For this review, take the finished solid that the model builds, in its own axes (mm). A direction names the side the tool comes from. Give positions to 0.01 mm unless a question says otherwise; leave off trailing zeros. Write each loop counter-clockwise with the first axis right and the second up, starting at its lowest first coordinate (ties: lowest second). Pieces come first, ordered by that corner, then holes. Notation, with made-up numbers: (30.25, 8) -> (40.25, 8) arc R20 cw to (40.25, 44) -> close; hole circle Ø10 at (24.25, -18.75). An arc over 180 degrees is marked (long way). Answer as CSV lines item,"result".
```python
from build123d import *

# Parameters (mm, degrees)
SKETCH1_R                = 100
BOSS_EXTRUDE1_DEPTH      = 10
SKETCH2_W                = 150
SKETCH2_H                = 150
BOSS_EXTRUDE2_DEPTH      = 20
FILLET1_R                = 20
SKETCH3_R                = 55
BOSS_EXTRUDE3_DEPTH      = 100
SKETCH4_R                = 65
BOSS_EXTRUDE4_DEPTH      = 10
SKETCH5_W                = 70
SKETCH5_H                = 90
BOSS_EXTRUDE5_DEPTH      = 90
CUT_EXTRUDE1_DEPTH       = 10
CHAMFER1_SIZE            = 10
SKETCH7_R                = 45
CUT_EXTRUDE2_DEPTH       = 100
BOSS_EXTRUDE6_DEPTH      = 10
SKETCH9_R                = 5
CUT_EXTRUDE3_DEPTH       = 2.5
FILLET9_R                = 5
CIRPATTERN1_COUNT        = 4
FILLET9_OF_CIRPATTERN1_R = 5


with BuildPart() as part:
    # Sketch1 → Boss-Extrude1 (new body)
    with BuildSketch(Plane(origin=(0, 0, 0), x_dir=(0, 0, -1), z_dir=(1, 0, 0))):
        Circle(SKETCH1_R)
    extrude(amount=BOSS_EXTRUDE1_DEPTH)

    # Sketch2 → Boss-Extrude2 (add)
    with BuildSketch(Plane(origin=(10, 0, 0), x_dir=(0, 0, -1), z_dir=(1, 0, 0))):
        Rectangle(SKETCH2_W, SKETCH2_H)
    extrude(amount=BOSS_EXTRUDE2_DEPTH)

    # Fillet1
    # the kernel refuses this fillet: 20 mm, written as the material it takes off along each edge
    with BuildSketch(Plane(origin=(10, -75, -75), x_dir=(0, 1, 0), z_dir=(1, 0, 0)), Plane(origin=(10, 75, 75), x_dir=(0, -1, 0), z_dir=(1, 0, 0)), Plane(origin=(10, -75, 75), x_dir=(0, 0, -1), z_dir=(1, 0, 0))) as fillet1_piece_1:
        with BuildLine():
            CenterArc((FILLET1_R, FILLET1_R), FILLET1_R, 180, 90)
            Line((0, FILLET1_R), (0, 0))
            Line((0, 0), (FILLET1_R, 0))
        make_face()
    extrude(amount=70, mode=Mode.SUBTRACT)
    with BuildSketch(Plane(origin=(10, 75, -75), x_dir=(0, -1, 0), z_dir=(1, 0, 0))) as fillet1_piece_2:
        with BuildLine():
            CenterArc((FILLET1_R, -FILLET1_R), FILLET1_R, 90, 90)
            Line((0, -FILLET1_R), (0, 0))
            Line((0, 0), (FILLET1_R, 0))
        make_face()
    extrude(amount=70, mode=Mode.SUBTRACT)

    # Sketch3 → Boss-Extrude3 (add)
    with BuildSketch(Plane(origin=(30, 0, 0), x_dir=(0, 0, -1), z_dir=(1, 0, 0))):
        with Locations(Location((0, 0, 0), (0, 0, 180))):
            Circle(SKETCH3_R)
    extrude(amount=BOSS_EXTRUDE3_DEPTH)

    # Sketch4 → Boss-Extrude4 (add)
    with BuildSketch(Plane(origin=(130, 0, 0), x_dir=(0, 0, -1), z_dir=(1, 0, 0))):
        Circle(SKETCH4_R)
    extrude(amount=BOSS_EXTRUDE4_DEPTH)

    # Sketch5 → Boss-Extrude5 (add)
    with BuildSketch(Plane.XY):
        with Locations((85, 0)):
            Rectangle(SKETCH5_W, SKETCH5_H)
    extrude(amount=BOSS_EXTRUDE5_DEPTH)

    # Sketch6 → Cut-Extrude1 (cut)
    with BuildSketch(Plane(origin=(120, 0, 0), x_dir=(0, 0, -1), z_dir=(1, 0, 0))):
        with BuildLine():
            Line((-90, -45), (-72.111025509, -45))
            ThreePointArc((-72.111025509, -45), (-85, 0), (-72.111025509, 45))
            Line((-72.111025509, 45), (-90, 45))
            Line((-90, 45), (-90, -45))
        make_face()
    extrude(amount=-CUT_EXTRUDE1_DEPTH, mode=Mode.SUBTRACT)

    # Chamfer1
    # the kernel refuses this chamfer: 10 mm, written as the material it adds along each edge
    with BuildSketch(Plane(origin=(110, 0, 0), x_dir=(0, -0.7581812704151473, 0.6520438337962206), z_dir=(0, -0.6520438337962206, -0.7581812704151473))) as chamfer1_piece_1_section:
        Polygon((85, -CHAMFER1_SIZE), (85 + CHAMFER1_SIZE, 0), (85, 0), align=None)
    chamfer1_piece_1 = revolve(axis=Axis((110, 0, 0), (-1, 0, 0)), revolution_arc=98.608247973, mode=Mode.PRIVATE)
    chamfer1_piece_1 = split(chamfer1_piece_1, bisect_by=Plane(origin=(118.167671654, 45, 80.674313719), z_dir=(0, -1, 0)), keep=Keep.TOP, mode=Mode.PRIVATE)
    chamfer1_piece_1 = split(chamfer1_piece_1, bisect_by=Plane(origin=(120, -31.470599687, 80.674313719), z_dir=(-1, 0, 0)), keep=Keep.TOP, mode=Mode.PRIVATE)
    chamfer1_piece_1 = split(chamfer1_piece_1, bisect_by=Plane(origin=(118.167671654, -45, 80.674313719), z_dir=(0, 1, 0)), keep=Keep.TOP, mode=Mode.PRIVATE)
    chamfer1_piece_1 = split(chamfer1_piece_1, bisect_by=Plane(origin=(118.167671654, -31.470599687, 90), z_dir=(0, 0, -1)), keep=Keep.TOP, mode=Mode.PRIVATE)
    add(chamfer1_piece_1)

    # Sketch7 → Cut-Extrude2 (cut)
    with BuildSketch(Plane(origin=(140, 0, 0), x_dir=(0, 0, -1), z_dir=(1, 0, 0))):
        Circle(SKETCH7_R)
    extrude(amount=-CUT_EXTRUDE2_DEPTH, mode=Mode.SUBTRACT)

    # Sketch8 → Boss-Extrude6 (add)
    with BuildSketch(Plane(origin=(30, 0, 0), x_dir=(0, 0, -1), z_dir=(1, 0, 0))):
        Polygon((67.320508076, -61.627449546), (67.320508076, -51.627449546), (58.660254038, -46.627449546), (50, -51.627449546), (50, -61.627449546), (58.660254038, -66.627449546), align=None)
    boss_extrude6 = extrude(amount=BOSS_EXTRUDE6_DEPTH)

    # Sketch9 → Cut-Extrude3 (cut)
    with BuildSketch(Plane(origin=(40, 0, 0), x_dir=(0, 0, -1), z_dir=(1, 0, 0))):
        with Locations((58.588222401, -56.525256823)):
            Circle(SKETCH9_R)
    cut_extrude3 = extrude(amount=-CUT_EXTRUDE3_DEPTH, mode=Mode.SUBTRACT)

    # Fillet9
    # the kernel refuses this fillet: 5 mm, written as the material it adds along each edge
    with BuildSketch(Plane(origin=(37.5, -56.525256823, -58.588222401), x_dir=(0, 0, -1), z_dir=(0, -1, 0))) as fillet9_piece_1:
        with BuildLine():
            CenterArc((0.669872981, 5), FILLET9_R, 270, 60)
            Line((0.669872981, 0), (0.669872981, -0.1))
            Line((0.669872981, -0.1), (5, -0.1))
            Line((5, -0.1), (5.1, 0))
            ThreePointArc((5.1, 0), (5.1, 1.25), (5.08660254, 2.45))
            Line((5.08660254, 2.45), (5, 2.5))
        make_face()
    revolve(axis=Axis((37.5, -56.525256823, -58.588222401), (1, 0, 0)))

    # CirPattern1: Boss-Extrude6, Cut-Extrude3 ×4 about axis
    cirpattern1_axis = Axis((0, 0, 0), (1, 0, 0))
    add([boss_extrude6.rotate(cirpattern1_axis, i * 360 / CIRPATTERN1_COUNT) for i in range(1, CIRPATTERN1_COUNT)])
    add([cut_extrude3.rotate(cirpattern1_axis, i * 360 / CIRPATTERN1_COUNT) for i in range(1, CIRPATTERN1_COUNT)], mode=Mode.SUBTRACT)

    # Fillet9 of CirPattern1
    # the kernel refuses this fillet: 5 mm, written as the material it adds along each edge
    with BuildSketch(Plane(origin=(37.5, 58.588222401, -56.525256823), x_dir=(0, 1, 0), z_dir=(0, 0, -1))) as fillet9_of_cirpattern1_piece_1:
        with BuildLine():
            CenterArc((0.669872981, 5), FILLET9_OF_CIRPATTERN1_R, 270, 60)
            Line((0.669872981, 0), (0.669872981, -0.1))
            Line((0.669872981, -0.1), (5, -0.1))
            Line((5, -0.1), (5.1, 0))
            ThreePointArc((5.1, 0), (5.1, 1.25), (5.08660254, 2.45))
            Line((5.08660254, 2.45), (5, 2.5))
        make_face()
    revolve(axis=Axis((37.5, 58.588222401, -56.525256823), (1, 0, 0)))
    with BuildSketch(Plane(origin=(37.5, 56.525256823, 58.588222401), x_dir=(0, 0, 1), z_dir=(0, 1, 0))) as fillet9_of_cirpattern1_piece_2:
        with BuildLine():
            CenterArc((0.669872981, 5), FILLET9_OF_CIRPATTERN1_R, 270, 60)
            Line((0.669872981, 0), (0.669872981, -0.1))
            Line((0.669872981, -0.1), (5, -0.1))
            Line((5, -0.1), (5.1, 0))
            ThreePointArc((5.1, 0), (5.1, 1.25), (5.08660254, 2.45))
            Line((5.08660254, 2.45), (5, 2.5))
        make_face()
    revolve(axis=Axis((37.5, 56.525256823, 58.588222401), (1, 0, 0)))
    with BuildSketch(Plane(origin=(37.5, -58.588222401, 56.525256823), x_dir=(0, -1, 0), z_dir=(0, 0, 1))) as fillet9_of_cirpattern1_piece_3:
        with BuildLine():
            CenterArc((0.669872981, 5), FILLET9_OF_CIRPATTERN1_R, 270, 60)
            Line((0.669872981, 0), (0.669872981, -0.1))
            Line((0.669872981, -0.1), (5, -0.1))
            Line((5, -0.1), (5.1, 0))
            ThreePointArc((5.1, 0), (5.1, 1.25), (5.08660254, 2.45))
            Line((5.08660254, 2.45), (5, 2.5))
        make_face()
    revolve(axis=Axis((37.5, -58.588222401, 56.525256823), (1, 0, 0)))


solid = part.part
```
Q1. Clearance check with flat-ended pins moving along their axes: pin 1 (6 mm diameter, centred on x = 20, y = 62.5, fed in from -Z); pin 2 (2 mm diameter, centred on x = 81.5, z = 69.5, fed in from +Y); pin 3 (1.5 mm diameter, centred on y = 74.5, z = 27, fed in from +X). State where each tip first meets the part, or that it passes through.
Answer block:
pin 1,"stops at z = -74.49"
pin 2,"stops at y = 45"
pin 3,"stops at x = 30"
Q2. To check wall thickness, follow probe 1 along Y at (x, z) = (114, 0); probe 2 along X at (y, z) = (-61, 3); probe 3 along Y at (x, z) = (9.5, -80.5). State the ranges of each line that lie inside material, in increasing order. Write a range as [from, to].
Answer block:
probe 1,"y = [-55, -45], [45, 55]"
probe 2,"x = [0, 30], [130, 140]"
probe 3,"y = [-59.33, 59.33]"
Q3. Add section A-A (x = 23). Write out the cut boundary in (y, z), plus the area to 3 significant figures.
Answer block:
outline,"(-75, -55) arc R20 ccw to (-55, -75) -> (55, -75) arc R20 ccw to (75, -55) -> (75, 55) arc R20 ccw to (55, 75) -> (-55, 75) arc R20 ccw to (-75, 55) -> close"
area,"22,200 mm2"
Q4. Add section B-B (y = 0). Write out the cut boundary in (x, z).
Answer block:
outline,"(0, -100) -> (10, -100) -> (10, -75) -> (30, -75) -> (30, -55) -> (130, -55) -> (130, -65) -> (140, -65) -> (140, -45) -> (40, -45) -> (40, 45) -> (140, 45) -> (140, 65) -> (130, 65) -> (130, 55) -> (120, 55) -> (120, 85) -> (115, 90) -> (50, 90) -> (50, 55) -> (30, 55) -> (30, 75) -> (10, 75) -> (10, 100) -> (0, 100) -> close"
Q5. Draft analysis for pull direction Z (two halves, no side actions). For faces 1 (the flat face through (34.93, 49.092, 54.391)), 2 (the flat face through (35, -57, -50)), 3 (the cylindrical face through (134.93, 19.52, -62)), 4 (the cylindrical face through (19.86, -68.986, 69.297)), state which applies: released by +Z, released by -Z, zero draft, split by the parting line, or undercut.
Answer block:
face 1,"undercut"
face 2,"undercut"
face 3,"split by the parting line"
face 4,"released by +Z"
Q6. Add section D-D (x = 90). Write out the cut boundary in (y, z).
Answer block:
outline,"(-45, 31.62) arc R55 ccw (long way) to (45, 31.62) -> (45, 90) -> (-45, 90) -> close; hole circle Ø90 at (0, 0)"
Q7. For faces 5 (the flat face through (34.93, -49.16, -63.05)), 6 (the flat face through (20, -1, 75)), 7 (the flat face through (83, 1, 90)), 8 (the flat face through (40, 1, 1)), list the 3-axis set-ups (+Z, -Z, +X, -X, +Y, -Y) from which the entire face can be reached by the end or side of a thin tool; tool diameter is ignored.
Answer block:
face 5,"-Z, +X"
face 6,"+Z, +Y, -Y"
face 7,"+Z, +X, +Y, -Y"
face 8,"+X"
Q8. Add section C-C (z = 0). Write out the cut boundary in (x, y).
Answer block:
outline,"(0, -100) -> (10, -100) -> (10, -75) -> (30, -75) -> (30, -55) -> (130, -55) -> (130, -65) -> (140, -65) -> (140, -45) -> (40, -45) -> (40, 45) -> (140, 45) -> (140, 65) -> (130, 65) -> (130, 55) -> (30, 55) -> (30, 75) -> (10, 75) -> (10, 100) -> (0, 100) -> close"
